from build123d import *

# Parameters (mm, degrees)
F0_R          = 30
F0_R_2        = 15
F1_DEPTH      = 5
F1_DEPTH_BACK = 5
F2_R          = 2.6556349186
F3_DEPTH      = 11.7


with BuildPart() as f1:
    # F0 (on Front) → F1 (new body, two sides)
    with BuildSketch(Plane.XZ) as f1_sk:
        Circle(F0_R)
        Circle(F0_R_2, mode=Mode.SUBTRACT)
    extrude(amount=F1_DEPTH)
    extrude(f1_sk.sketch, amount=-F1_DEPTH_BACK)

    # F2
    f2_edges = [f1.edges().sort_by_distance(p)[0] for p in [
        (-30, -5, 0),
        (-15, -5, 0),
    ]]
    fillet(f2_edges, radius=F2_R)

    # F3 (add): a face of the model
    f3_faces = [f1.faces().sort_by_distance(p)[0] for p in [
        (-26.5709496423, -5, 0),
    ]]
    extrude(f3_faces, amount=F3_DEPTH)


solid = f1.part
Verification items for the finished model (mm, model axes). A direction names the side the tool comes from. Coordinates: 2 decimals unless noted, no trailing zeros. Write each loop counter-clockwise with the first axis right and the second up, starting at its lowest first coordinate (ties: lowest second). Pieces come first, ordered by that corner, then holes. Notation, with made-up numbers: M 75.25,37 L 84.25,37 A13 cw 84.25,55 Z; hole C 67.25,57.5 d9. An arc over 180 degrees is marked long. Use a Markdown table: item, result.
Q1. Set-up check for faces 4 (the face through (-5.9, -10.8, -26.7)), 5 (the face through (6, 5, 14)): record each of +Z, -Z, +X, -X, +Y, -Y from which the full face is reachable in a straight line by a thin tool's end or side.
Reply:
| item | result |
|---|---|
| face 4 | -Y |
| face 5 | +Z, -Z, +X, -X, +Y |
Q2. Thickness scan on line 1 (Z direction, x = 0, y = -1.2); line 2 (Z direction, x = 0, y = -9.5); line 3 (X direction, y = -14, z = 4). Record the ranges inside material, lowest first.
Reply:
| item | result |
|---|---|
| line 1 | z = -30 to -15, 15 to 30 |
| line 2 | z = -27.34 to -17.66, 17.66 to 27.34 |
| line 3 | x = -27.05 to -17.2, 17.2 to 27.05 |
Q3. Sectioned sample at B-B, the plane z = 0. Record the boundary of the cut face in (x, y).
Reply:
| item | result |
|---|---|
| outline | M -30,-2.34 A2.66 ccw -27.34,-5 L -27.34,-16.7 L -17.66,-16.7 L -17.66,-5 A2.66 ccw -15,-2.34 L -15,5 L -30,5 Z; M 15,-2.34 A2.66 ccw 17.66,-5 L 17.66,-16.7 L 27.34,-16.7 L 27.34,-5 A2.66 ccw 30,-2.34 L 30,5 L 15,5 Z |
Q4. Sectioned sample at D-D, the plane y = -12.5. Record the boundary of the cut face in (x, z).
Reply:
| item | result |
|---|---|
| outline | C 0,0 d54.69; hole C 0,0 d35.31 |
Q5. Go/stop test with flat-tipped pins: P1, Ø6, axis at x = -22, y = -7.5, coming from the -Z side; P2, Ø1.5, axis at x = 6.5, y = 2, coming from the +Z side; P3, Ø18, axis at x = 0, z = 0, coming from the +Y side; P4, Ø6, axis at x = 13.5, y = -9, coming from the +Z side. Record where each tip stops, or that it passes through.
Reply:
| item | result |
|---|---|
| P1 | stops at z = -19.67 |
| P2 | stops at z = 29.44 |
| P3 | passes through |
| P4 | stops at z = 25.25 |
Q6. Draft check along Z on faces 1 (the face through (-29.97, 1.28, 1.32)), 2 (the face through (0, -16.7, -18)), 3 (the face through (16.84, -10.77, 5.3)). Enter one of: +Z half, -Z half, draft (parallel to the pull), parting line (faces both ways), or undercut.
Reply:
| item | result |
|---|---|
| face 1 | parting line |
| face 2 | draft |
| face 3 | undercut |
Q7. Sectioned sample at C-C, the plane y = 3.5. Record the boundary of the cut face in (x, z).
Reply:
| item | result |
|---|---|
| outline | C 0,0 d60; hole C 0,0 d30 |
Q8. Sectioned sample at A-A, the plane x = 0. Record the boundary of the cut face in (y, z).
Reply:
| item | result |
|---|---|
| outline | M -16.7,-27.34 L -5,-27.34 A2.66 ccw -2.34,-30 L 5,-30 L 5,-15 L -2.34,-15 A2.66 ccw -5,-17.66 L -16.7,-17.66 Z; M -16.7,17.66 L -5,17.66 A2.66 ccw -2.34,15 L 5,15 L 5,30 L -2.34,30 A2.66 ccw -5,27.34 L -16.7,27.34 Z |
